Geometry check sheet. Reference: the model listing, model coordinates, mm. Face numbers are marked on the shaded views. A direction names the side the tool comes from. Round coordinates to 2 decimals unless told otherwise and drop trailing zeros. Write each loop counter-clockwise with the first axis right and the second up, starting at its lowest first coordinate (ties: lowest second). Pieces come first, ordered by that corner, then holes. Notation, with made-up numbers: M 16.5,85.5 L 35.5,85.5 A34 ccw 35.5,120.5 Z; hole C 71.5,-31.75 d4. An arc over 180 degrees is marked long. Put each result on its own line as item: value. Start each with the question number.
(1) Section check B-B on z = 12.5. Record the cut outline in (x, y).
(2) Gauge pin test, flat ends, axial feed: pin 1 (5 mm diameter, centred on x = -16.5, z = 53, fed in from -Y); pin 2 (4 mm diameter, centred on x = 17, z = 60.5, fed in from -Y). Record the tip position at first contact, or that the pin passes through.
(3) Material ranges on probe 1 along Z at (x, y) = (-18.5, 22.5); probe 2 along Y at (x, z) = (17.5, 50); probe 3 along X at (y, z) = (-16.5, 63.5), recorded low to high.
(4) Section check A-A on y = 0. Record the cut outline in (x, z) (3 decimals).
(5) Section check C-C on z = 52.5. Record the cut outline in (x, y).
(6) Tool access check on the marked faces 1 and 2. Record the directions out of +Z, -Z, +X, -X, +Y, -Y that give a thin tool (end or side, any length) a straight path to the whole face; none if there is none.
Autodesk Inventor part; units mm, degrees
ref_plane "YZ Plane" through (0, 0, 0) normal (1, 0, 0) x (0, 1, 0)
ref_plane "XZ Plane" through (0, 0, 0) normal (0, 1, 0) x (-1, 0, 0)
ref_plane "XY Plane" through (0, 0, 0) normal (0, 0, 1) x (1, 0, 0)
sketch "Sketch1" plane through (0, 0, 0) normal (0, 0, 1) x (1, 0, 0)
  line L0 (-35, 0) -> (35, 0)
  line L1 (0, -35) -> (0, 35)
  line L2 (-25, 25) -> (25, 25)
  line L3 (25, 25) -> (25, -25)
  line L4 (25, -25) -> (-25, -25)
  line L5 (-25, -25) -> (-25, 25)
  point P0 (0, 0)
  point P1 (-25, 0)
  point P2 (0, 25)
  dimension "d0" = 50
extrude "Extrusion1" add sketch "Sketch1" along normal blind 41
sketch "Sketch2" plane through (0, 0, 41) normal (0, 0, 1) x (1, 0, 0)
  circle A0 centre (0, 0) radius 22.225
  dimension "d3" = 44.45
extrude "Extrusion2" add sketch "Sketch2" along normal blind 28.5 draft -5
fillet "Fillet1" radius 12.7 4 edges at (25, 25, 20.5) (25, -25, 20.5) (-25, 25, 20.5) (-25, -25, 20.5)
properties part number "rangefinder model"
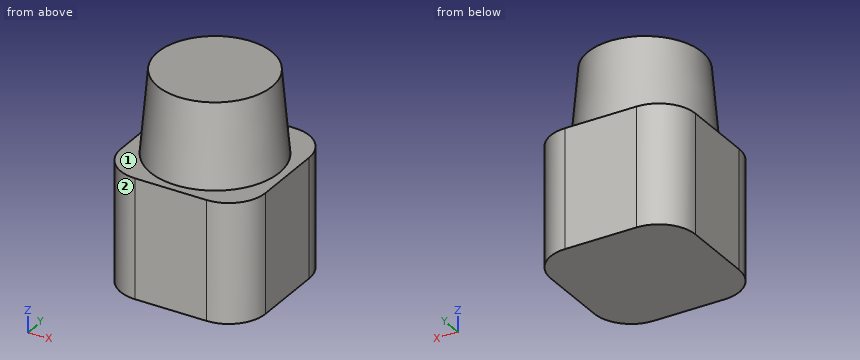
Answers follow:
1. outline: M -25,-12.3 A12.7 ccw -12.3,-25 L 12.3,-25 A12.7 ccw 25,-12.3 L 25,12.3 A12.7 ccw 12.3,25 L -12.3,25 A12.7 ccw -25,12.3 Z
2. pin 1: stops at y = -15.91
2. pin 2: stops at y = -14.02
3. probe 1: z = 0 to 41
3. probe 2: y = -12.38 to 12.38
3. probe 3: x = -11.75 to 11.75
4. outline: M -25,0 L 25,0 L 25,41 L 22.225,41 L 19.732,69.5 L -19.732,69.5 L -22.225,41 L -25,41 Z
5. outline: C 0,0 d42.44
6. face 1: +Z
6. face 2: +Z, -Z, -X, -Y
